The listing builds one solid part. Answer for the finished solid, in the listing's coordinates (mm). A direction names the side the tool comes from. Coordinates: 2 decimals unless noted, no trailing zeros. Loops run counter-clockwise (first coordinate to the right, second up) from the corner with the lowest first, then second, coordinate; pieces in that order, holes last. Notation, with made-up numbers: M -21.5,-17.75 L 33.5,-17.75 A27 ccw 33.5,8.25 Z; hole C -28.5,38 d1. An arc over 180 degrees is marked long. Return JSON: item names as keys, results as strings. Group by question number.
1. Section B-B (z = 0) is taken. Write down the section's boundary in (x, y), then the cut area to 3 significant figures.
2. Given P1, Ø2, axis at x = 0.5, y = 23, coming from the +Z side; P2, Ø1.5, axis at y = 26, z = 2.5, coming from the +X side; P3, Ø3, axis at x = 2.5, y = 8, coming from the -Z side, each flat-ended and moving along its own axis, determine where each tip first touches the part or whether it passes through.
3. Section C-C (y = 23.5) is taken. Write down the section's boundary in (x, z).
4. Section A-A (x = 0) is taken. Write down the section's boundary in (y, z).
5. Which of the six approach directions +Z, -Z, +X, -X, +Y, -Y give full straight-line access (tool end or side, diameter ignored) to faces 1 (the face through (4.88, 19.03, -1.08)), 2 (the face through (-3.955, 0.986, -5.158))?
6. Straight lines are drawn through the part: L1, parallel to X at y = 16.5, z = -0.25; L2, parallel to X at y = 26, z = 2.75. For each, find the intervals that lie inside material, in ascending order. Write a range as from..to.
```python
from build123d import *

# Parameters (mm, degrees)
SKETCH_1_R          = 6.5
EXTRUDE_1_DEPTH     = 35
CUT_EXTRUDE_START   = -30
SKETCH_2_R          = 6.5
SKETCH_2_R_2        = 5
CUT_EXTRUDE_1_DEPTH = 30
CHAMFER_1_SIZE      = 3


with BuildPart() as part:
    # Эскиз1 → Бобышка-Вытянуть1 (new body)
    with BuildSketch(Plane(origin=(0, 0, 0), x_dir=(1, 0, 0), z_dir=(0, 1, 0))):
        with Locations(Location((0, 0, 0), (0, 0, 270))):
            Circle(SKETCH_1_R)
    extrude(amount=EXTRUDE_1_DEPTH)

    # Эскиз2 → Вырез-Вытянуть1 (cut)
    with BuildSketch(Plane(origin=(0, 35, 0), x_dir=(1, 0, 0), z_dir=(0, 1, 0)).offset(CUT_EXTRUDE_START)):
        with Locations(Location((0, 0, 0), (0, 0, 270))):
            Circle(SKETCH_2_R)
        with Locations(Location((0, 0, 0), (0, 0, 270))):
            Circle(SKETCH_2_R_2, mode=Mode.SUBTRACT)
    extrude(amount=CUT_EXTRUDE_1_DEPTH, mode=Mode.SUBTRACT)

    # Фаска1
    # the kernel refuses this chamfer: 3 mm, written as the material it takes off along each edge
    with BuildSketch(Plane(origin=(0, 5, 0), x_dir=(0, 0, 1), z_dir=(-1, 0, 0))) as chamfer_1_piece_1_section:
        Polygon((6.5, -CHAMFER_1_SIZE), (6.5 - CHAMFER_1_SIZE, 0), (6.5, 0), align=None)
    chamfer_1_piece_1 = revolve(axis=Axis((0, 5, 0), (0, 1, 0)), mode=Mode.PRIVATE)
    chamfer_1_piece_1 = chamfer_1_piece_1 - Plane(origin=(0, 2.743926997, 0), x_dir=(0, 0, 1), z_dir=(0, -1, 0)) * Cylinder(5, 27, mode=Mode.PRIVATE)
    add(chamfer_1_piece_1, mode=Mode.SUBTRACT)


solid = part.part
```
Worked out:
{
 "1": {"outline": "M -6.5,0 L 6.5,0 L 6.5,2 L 5,3.5 L 5,35 L -5,35 L -5,3.5 L -6.5,2 Z", "area": "358 mm^2"},
 "2": {"P1": "z = 5", "P2": "x = 4.68", "P3": "z = -4.9"},
 "3": {"outline": "C 0,0 d10"},
 "4": {"outline": "M 0,-6.5 L 2,-6.5 L 3.5,-5 L 35,-5 L 35,5 L 3.5,5 L 2,6.5 L 0,6.5 Z"},
 "5": {"face 1": "+Y", "face 2": "+Y, -Y"},
 "6": {"L1": "-4.99..4.99", "L2": "-4.18..4.18"}
}
